Can you work these out from the drawing? Everything is in mm from the part's minimum corner. Coordinates: 2 decimals unless noted, no trailing zeros. Loops run counter-clockwise (first coordinate to the right, second up) from the corner with the lowest first, then second, coordinate; pieces in that order, holes last. Notation, with made-up numbers: M 81.5,-38 L 88.5,-38 A13 ccw 88.5,-26 Z; hole C 17,28.25 d7. An arc over 180 degrees is marked long. Use CSV: the item, a comma, the result in double quotes. Start each with the question number.
Q1. If we section it at D-D (z = 60): Please give me the cut outline in (x, y), and give its area (3 significant figures).
Q2. Please list where these lines run through material, in increasing order: probe 1 along X at (y, z) = (1.5, 30); probe 2 along Z at (x, y) = (67.5, 2.1); probe 3 along X at (y, z) = (2.5, 11). Write a range as [from, to].
Q3. If we section it at A-A (z = 70): Please give me the cut outline in (x, y).
Q4. For pin 1 Ø0.9 at (x, y) = (46.5, 1) entering from -Z; pin 2 Ø1.5 at (x, z) = (42.5, 9.5) entering from +Y; pin 3 Ø1.5 at (x, y) = (1, 1.5) entering from -Z, each with a flat end and sliding along its axis, tell me the tip position at first contact or that it passes through.
Q5. If we section it at B-B (x = 22.5): Please give me the cut outline in (y, z).
Q6. If we section it at C-C (y = 0.95): State how many separate pieces and enclosed holes the cut face has, and give its area (3 significant figures).
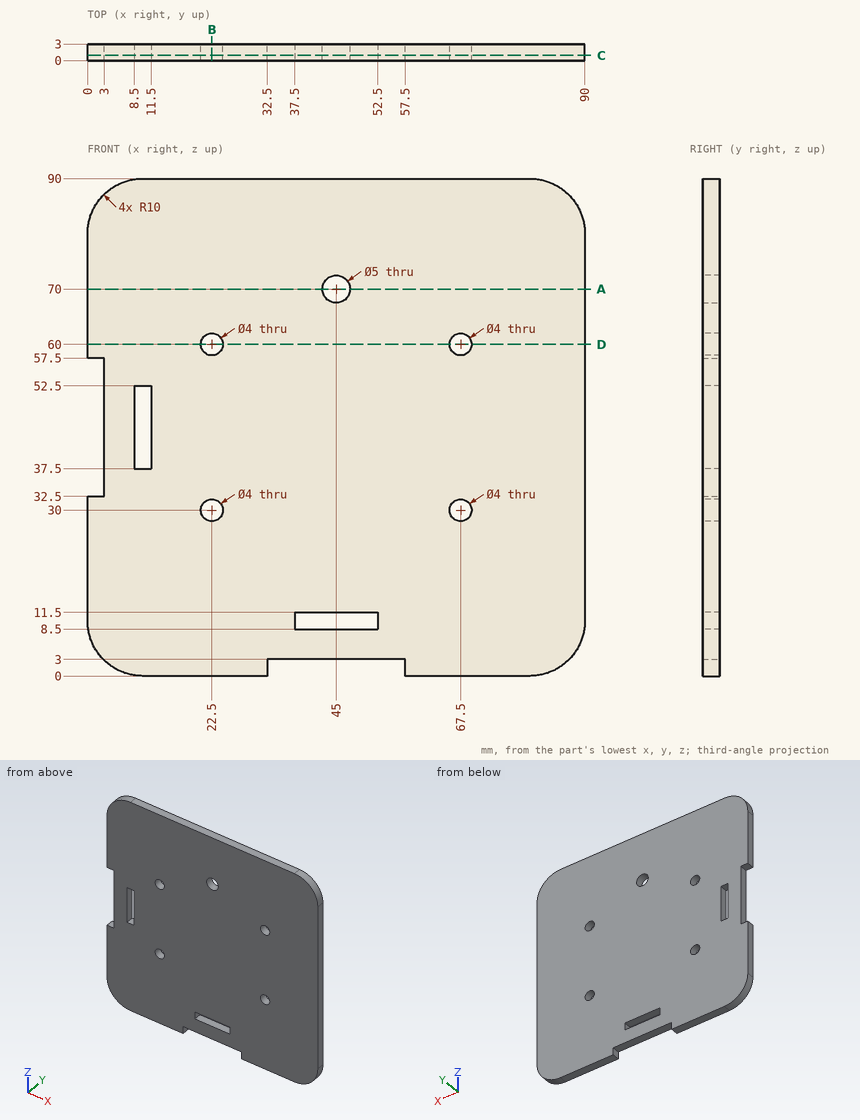
Results below:
1,outline,"M 0,0 L 20.5,0 L 20.5,3 L 0,3 Z; M 24.5,0 L 65.5,0 L 65.5,3 L 24.5,3 Z; M 69.5,0 L 90,0 L 90,3 L 69.5,3 Z"
1,area,"246 mm^2"
2,probe 1,"[0, 20.5], [24.5, 65.5], [69.5, 90]"
2,probe 2,"[0, 28], [32, 58], [62, 90]"
2,probe 3,"[0, 37.5], [52.5, 90]"
3,outline,"M 0,0 L 42.5,0 L 42.5,3 L 0,3 Z; M 47.5,0 L 90,0 L 90,3 L 47.5,3 Z"
4,pin 1,"z = 3"
4,pin 2,"through"
4,pin 3,"z = 4.35"
5,outline,"M 0,0 L 3,0 L 3,28 L 0,28 Z; M 0,32 L 3,32 L 3,58 L 0,58 Z; M 0,62 L 3,62 L 3,90 L 0,90 Z"
6,separate pieces,"1"
6,enclosed holes,"7"
6,area,"7,700 mm^2"
